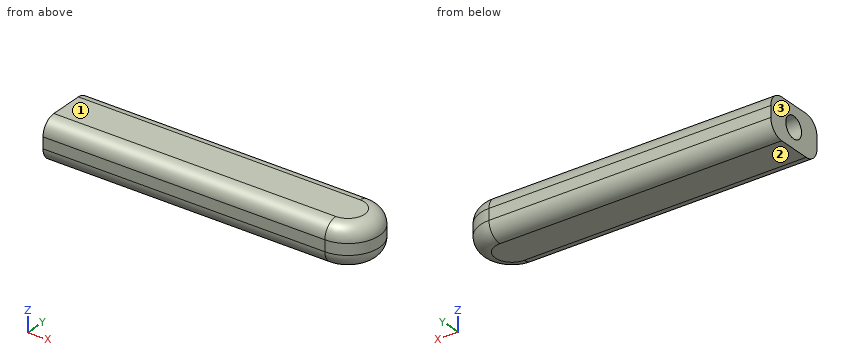
from build123d import *

# Parameters (mm, degrees)
F1_DEPTH = 11
F2_R     = 4
F3_R     = 4
F4_R     = 2.888832
F5_DEPTH = 65


with BuildPart() as f1:
    # F0 (on Top) → F1 (new body)
    with BuildSketch(Plane.XY):
        with BuildLine():
            Line((35.975721, 11.224424), (-40.004998, 11.224424))
            Line((-40.004998, 11.224424), (-40.004998, -5.756116))
            Line((-40.004998, -5.756116), (35.975721, -5.756116))
            ThreePointArc((35.975721, -5.756116), (44.465991, 2.734154), (35.975721, 11.224424))
        make_face()
    extrude(amount=F1_DEPTH)

    # F2
    f2_edges = [f1.edges().sort_by_distance(p)[0] for p in [
        (-2.014639, -5.756116, 11),
        (44.465991, 2.734154, 11),
        (-2.014639, 11.224424, 11),
    ]]
    fillet(f2_edges, radius=F2_R)

    # F3
    f3_edges = [f1.edges().sort_by_distance(p)[0] for p in [
        (-2.014639, 11.224424, 0),
        (-2.014639, -5.756116, 0),
        (44.465991, 2.734154, 0),
    ]]
    fillet(f3_edges, radius=F3_R)

    # F4 (on face) → F5 (cut)
    with BuildSketch(Plane(origin=(-40.004998, 0, 0), x_dir=(0, -1, 0), z_dir=(-1, 0, 0))):
        with Locations((-2.832736, 5.382194)):
            Circle(F4_R)
    extrude(amount=-F5_DEPTH, mode=Mode.SUBTRACT)


solid = f1.part
Can you work these out from the model? Positions are in its coordinate system, mm. Face numbers are marked on the shaded views. Give positions to 0.01 mm unless a question says otherwise; leave off trailing zeros. Write each loop counter-clockwise with the first axis right and the second up, starting at its lowest first coordinate (ties: lowest second). Pieces come first, ordered by that corner, then holes. Notation, with made-up numbers: (10, -31) -> (65, -31) arc R14 cw to (65, -12) -> close; hole circle Ø7 at (-32.5, 78.25). An arc over 180 degrees is marked (long way). Answer as a JSON object with one key per item and string values. Group by question number.
Item 1: I'm going to push flat-ended pins straight in: P1, Ø2, axis at x = 22, y = 9, coming from the +Z side; P2, Ø3, axis at y = 3.5, z = 5, coming from the -X side (3 decimals); P3, Ø6, axis at y = -2.5, z = 3.5, coming from the +X side. Where does each tip first touch, or does it pass through?
Item 2: Suppose I cut it at A-A (x = 21). Please give me the cut outline in (y, z), plus the area to 3 significant figures.
Item 3: We'd pull the mould along Z, two halves only. Please class the marked faces 1, 2 and 3: +Z half, -Z half, draft (parallel to the pull), parting line (faces both ways), or undercut.
Item 4: Suppose I cut it at C-C (z = 1.5). Please give me the cut outline in (x, y) (3 decimals), plus the area to 3 significant figures.
Item 5: Please list where these lines run through material, in increasing order: line 1 (Y direction, x = 17, z = 5.5); line 2 (Z direction, x = 3.5, y = 4.5); line 3 (Y direction, x = -10, z = 3). Write a range as [from, to].
Item 6: Suppose I cut it at B-B (z = 10.25). Please give me the cut outline in (x, y) (3 decimals), plus the area to 3 significant figures.
Findings:
{
 "1": {"P1": "stops at z = 10.92", "P2": "stops at x = 24.995", "P3": "stops at x = 44.16"},
 "2": {"outline": "(-5.76, 4) arc R4 ccw to (-1.76, 0) -> (7.22, 0) arc R4 ccw to (11.22, 4) -> (11.22, 7) arc R4 ccw to (7.22, 11) -> (-1.76, 11) arc R4 ccw to (-5.76, 7) -> close; hole circle Ø5.78 at (2.83, 5.38)", "area": "147 mm²"},
 "3": {"face 1": "+Z half", "face 2": "-Z half", "face 3": "draft"},
 "4": {"outline": "(-40.005, -4.879) -> (35.976, -4.879) arc R7.613 ccw to (35.976, 10.347) -> (-40.005, 10.347) -> close", "area": "1,250 mm²"},
 "5": {"line 1": "y = [-5.76, -0.05], [5.72, 11.22]", "line 2": "z = [0, 3.02], [7.74, 11]", "line 3": "y = [-5.63, 1.2], [4.47, 11.1]"},
 "6": {"outline": "(-40.005, -4.088) -> (35.976, -4.088) arc R6.822 ccw to (35.976, 9.556) -> (-40.005, 9.556) -> close", "area": "1,110 mm²"}
}
